Work out the finished part from the listing and answer in its coordinate system (mm). Coordinates: 2 decimals unless noted, no trailing zeros. Loops run counter-clockwise (first coordinate to the right, second up) from the corner with the lowest first, then second, coordinate; pieces in that order, holes last. Notation, with made-up numbers: (76.25, 27) -> (112.25, 27) arc R11 cw to (112.25, 46) -> close; hole circle Ø8 at (83, 71.25). An arc over 180 degrees is marked (long way). Use a Markdown table: item, result. Add a question column.
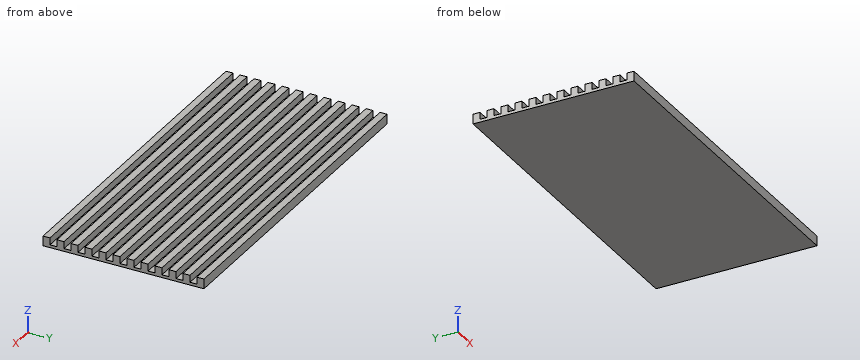
```python
from build123d import *

# Parameters (mm, degrees)
SKETCH_1_W             = 2400
SKETCH_1_H             = 1150
EXTRUDE_1_DEPTH        = 20
SKETCH_2_W             = 2400
SKETCH_2_H             = 50
EXTRUDE_2_DEPTH        = 50
PATTERN_LINEAR_1_COUNT = 12
PATTERN_LINEAR_1_PITCH = 100


with BuildPart() as part:
    # Эскиз1 → Бобышка-Вытянуть1 (new body)
    with BuildSketch(Plane.XY):
        with Locations((1200, 575)):
            Rectangle(SKETCH_1_W, SKETCH_1_H)
    extrude(amount=EXTRUDE_1_DEPTH)

    # Эскиз2 → Бобышка-Вытянуть2 (add)
    with BuildSketch(Plane.XY.offset(20)):
        with Locations((1200, 1125)):
            Rectangle(SKETCH_2_W, SKETCH_2_H)
    extrude_2 = extrude(amount=EXTRUDE_2_DEPTH)

    # Линейный массив1: Бобышка-Вытянуть2 ×12
    with Locations(*[(0, -i * PATTERN_LINEAR_1_PITCH, 0) for i in range(1, PATTERN_LINEAR_1_COUNT)]):
        add(extrude_2)


solid = part.part
```
Item 1: Given pin 1 (8 mm diameter, centred on x = 1527.5, y = 1029, fed in from -Z); pin 2 (25 mm diameter, centred on x = 1584.5, y = 1070, fed in from +Z), each flat-ended and moving along its own axis, determine where each tip first touches the part or whether it passes through.
Item 2: Find the intervals of material crossed by probe 1 along Z at (x, y) = (2240, 964), in increasing order.
Item 3: Section A-A (z = 59.5) is taken. Count the separate pieces of the cut face and the enclosed holes in it, then the cut area to 3 significant figures.
Item 4: Section B-B (y = 1071.5) is taken. Determine the outline of the cut face in (x, z), then the cut area to 3 significant figures.
Output:
| question | item | result |
|---|---|---|
| 1 | pin 1 | stops at z = 0 |
| 1 | pin 2 | stops at z = 20 |
| 2 | probe 1 | z = 0 to 20 |
| 3 | separate pieces | 12 |
| 3 | enclosed holes | 0 |
| 3 | area | 1,440,000 mm2 |
| 4 | outline | (0, 0) -> (2400, 0) -> (2400, 20) -> (0, 20) -> close |
| 4 | area | 48,000 mm2 |
